Part model, mm, in its own coordinate system. Round coordinates to 2 decimals unless told otherwise and drop trailing zeros. Loops run counter-clockwise (first coordinate to the right, second up) from the corner with the lowest first, then second, coordinate; pieces in that order, holes last.
(1) Cut at C-C on x = 17.5. List the corners of the cut face in (y, z).
(2) Flat gauge pin, fed straight in: pin 1 (1.6 mm diameter, centred on x = 0, y = -23.5, fed in from +Z). Where does the tip first touch, or does it go through?
(3) Cut at B-B on y = -23.5. List the corners of the cut face in (x, z).
(4) Cut at D-D on z = 1.05. Count the separate pieces of the cut face and the enclosed holes in it, then the cut area to 3 significant figures.
(5) Probe probe 1 along Y at (x, z) = (0, 1.05); probe 2 along Y at (x, z) = (17.5, 0.7); probe 3 along Y at (x, z) = (17, 0.8). List the from-to ranges inside material, lowest first.
(6) Cut at A-A on x = 0. List the corners of the cut face in (y, z), then the cut area to 3 significant figures.
from build123d import *

# Parameters (mm, degrees)
SKETCH_1_R          = 1
SKETCH_1_R_2        = 5
EXTRUDE_1_DEPTH     = 1.5
SKETCH_3_R          = 1
CUT_EXTRUDE_1_DEPTH = 10
FILLET_1_R          = 3


with BuildPart() as part:
    # 草图1 → 凸台-拉伸1 (new body)
    with BuildSketch(Plane.XY):
        Polygon((7.5, 22.5), (-7.5, 22.5), (-7.5, -27.5), (7.5, -27.5), (27.5, -27.5), (27.5, 2.5), (27.5, 14.5), (27.5, 22.5), (27.5, 28.5), (7.5, 28.5), align=None)
        with Locations((0, -23.5)):
            Circle(SKETCH_1_R, mode=Mode.SUBTRACT)
        with Locations((0, 16.5)):
            Circle(SKETCH_1_R, mode=Mode.SUBTRACT)
        with Locations((17.5, 16.5)):
            Circle(SKETCH_1_R_2, mode=Mode.SUBTRACT)
    extrude(amount=EXTRUDE_1_DEPTH)

    # 草图3 → 切除-拉伸1 (cut)
    with BuildSketch(Plane.XY.offset(1.5)):
        with Locations((17.5, -2.8)):
            Circle(SKETCH_3_R)
        with Locations((17.5, 25)):
            Circle(SKETCH_3_R)
    extrude(amount=-CUT_EXTRUDE_1_DEPTH, mode=Mode.SUBTRACT)

    # 圆角1
    fillet_1_edges = [part.edges().sort_by_distance(p)[0] for p in [
        (7.5, 22.5, 0.75),
        (7.5, 28.5, 0.75),
        (-7.5, 22.5, 0.75),
        (27.5, 28.5, 0.75),
        (-7.5, -27.5, 0.75),
        (27.5, -27.5, 0.75),
    ]]
    fillet(fillet_1_edges, radius=FILLET_1_R - 0.0001)  # a hair under: the kernel refuses the full size


solid = part.part
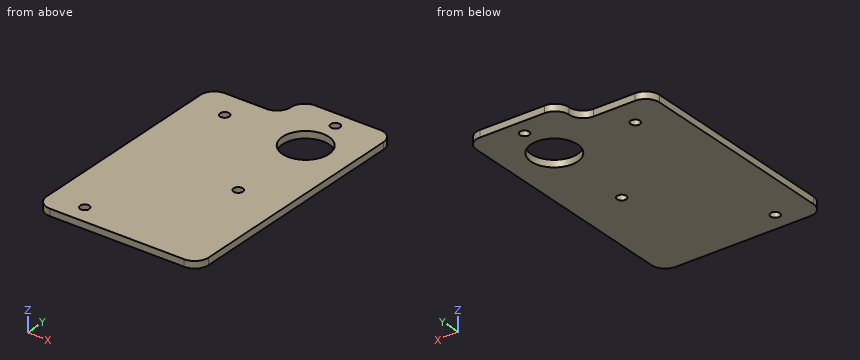
Final values:
1. outline: (-27.5, 0) - (-3.8, 0) - (-3.8, 1.5) - (-27.5, 1.5) - close; (-1.8, 0) - (11.5, 0) - (11.5, 1.5) - (-1.8, 1.5) - close; (21.5, 0) - (24, 0) - (24, 1.5) - (21.5, 1.5) - close; (26, 0) - (28.5, 0) - (28.5, 1.5) - (26, 1.5) - close
2. pin 1: passes through
3. outline: (-7.5, 0) - (-1, 0) - (-1, 1.5) - (-7.5, 1.5) - close; (1, 0) - (27.5, 0) - (27.5, 1.5) - (1, 1.5) - close
4. separate pieces: 1
4. enclosed holes: 5
4. area: 1,770 mm2
5. probe 1: y = -27.5 to -24.5, -22.5 to 15.5, 17.5 to 22.5
5. probe 2: y = -27.5 to -3.8, -1.8 to 11.5, 21.5 to 24, 26 to 28.5
5. probe 3: y = -27.5 to -3.67, -1.93 to 11.53, 21.47 to 24.13, 25.87 to 28.5
6. outline: (-27.5, 0) - (-24.5, 0) - (-24.5, 1.5) - (-27.5, 1.5) - close; (-22.5, 0) - (15.5, 0) - (15.5, 1.5) - (-22.5, 1.5) - close; (17.5, 0) - (22.5, 0) - (22.5, 1.5) - (17.5, 1.5) - close
6. area: 69.0 mm2
